Design review of the part built by this model. Coordinates are the model's own, in mm. Coordinates: 2 decimals unless noted, no trailing zeros. Order: outer loops, then holes, each group sorted by start corner. A loop starts at its lowest first (then second) coordinate and runs counter-clockwise, first axis right, second up. Notation, with made-up numbers: M -11.75,75 L 30.25,75 A23 ccw 30.25,109 Z; hole C 59,-28 d5. An arc over 180 degrees is marked long. Answer as a JSON object with one key per item and string values.
from build123d import *

# Parameters (mm, degrees)
BOSS_EXTRUDE1_DEPTH = 8
CUT_EXTRUDE1_DEPTH  = 200.784047411


with BuildPart() as part:
    # Sketch1 → Boss-Extrude1 (new body)
    with BuildSketch(Plane(origin=(0, 0, 0), x_dir=(1, 0, 0), z_dir=(0, 1, 0))):
        Polygon((8, 117.16), (0, 117.16), (0, 30), (8, 30), (8, 0), (92, 0), (92, 30), (100, 30), (100, 117.16), (92, 117.16), (92, 177.16), (8, 177.16), align=None)
    extrude(amount=BOSS_EXTRUDE1_DEPTH)

    # Sketch2 → Cut-Extrude1 (cut, through all)
    with BuildSketch(Plane.ZY.offset(-8)):
        Polygon((0, 8), (-8, 0), (0, 0), align=None)
    extrude(amount=-CUT_EXTRUDE1_DEPTH, mode=Mode.SUBTRACT)


solid = part.part
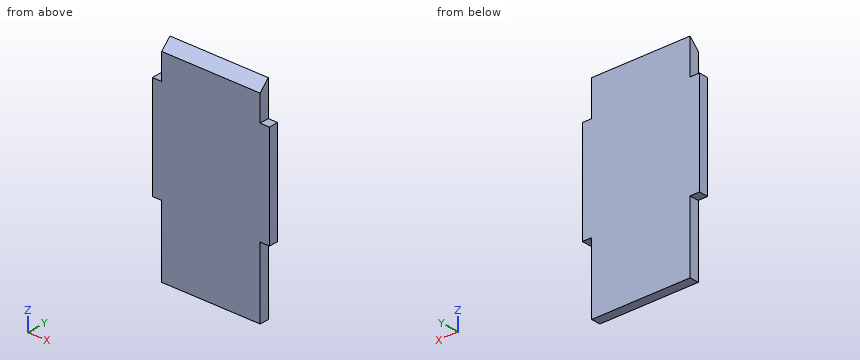
1) Add section B-B (z = -19.5). State the section outline as (x, y) points.
Taken from the geometry:
{"outline": "M 8,0 L 92,0 L 92,8 L 8,8 Z"}
2) To check wall thickness, follow L1, parallel to X at y = 1.5, z = -163; L2, parallel to Z at x = 95, y = 2.5; L3, parallel to Z at x = 32, y = 2.75. State the ranges of each line that lie inside material, in increasing order.
Taken from the geometry:
{"L1": "x = 8 to 92", "L2": "z = -117.16 to -30", "L3": "z = -177.16 to -5.25"}
3) Add section A-A (y = 6). State the section outline as (x, z) points, and give its area (3 significant figures).
Taken from the geometry:
{"outline": "M 0,-117.16 L 8,-117.16 L 8,-177.16 L 92,-177.16 L 92,-117.16 L 100,-117.16 L 100,-30 L 92,-30 L 92,-2 L 8,-2 L 8,-30 L 0,-30 Z", "area": "16,100 mm2"}
4) Insertion check: pin 1 Ø2.5 at (y, z) = (2.5, -21.5) entering from +X; pin 2 Ø4 at (y, z) = (3, -22) entering from -X; pin 3 Ø4 at (x, y) = (4, 5.5) entering from +Z. Each pin has a flat end and moves straight along its axis. Give the tip position at first contact, or say it passes through.
Taken from the geometry:
{"pin 1": "stops at x = 92", "pin 2": "stops at x = 8", "pin 3": "stops at z = -30"}
5) Add section C-C (x = 54.5). State the section outline as (y, z) points.
Taken from the geometry:
{"outline": "M 0,-177.16 L 8,-177.16 L 8,0 L 0,-8 Z"}
